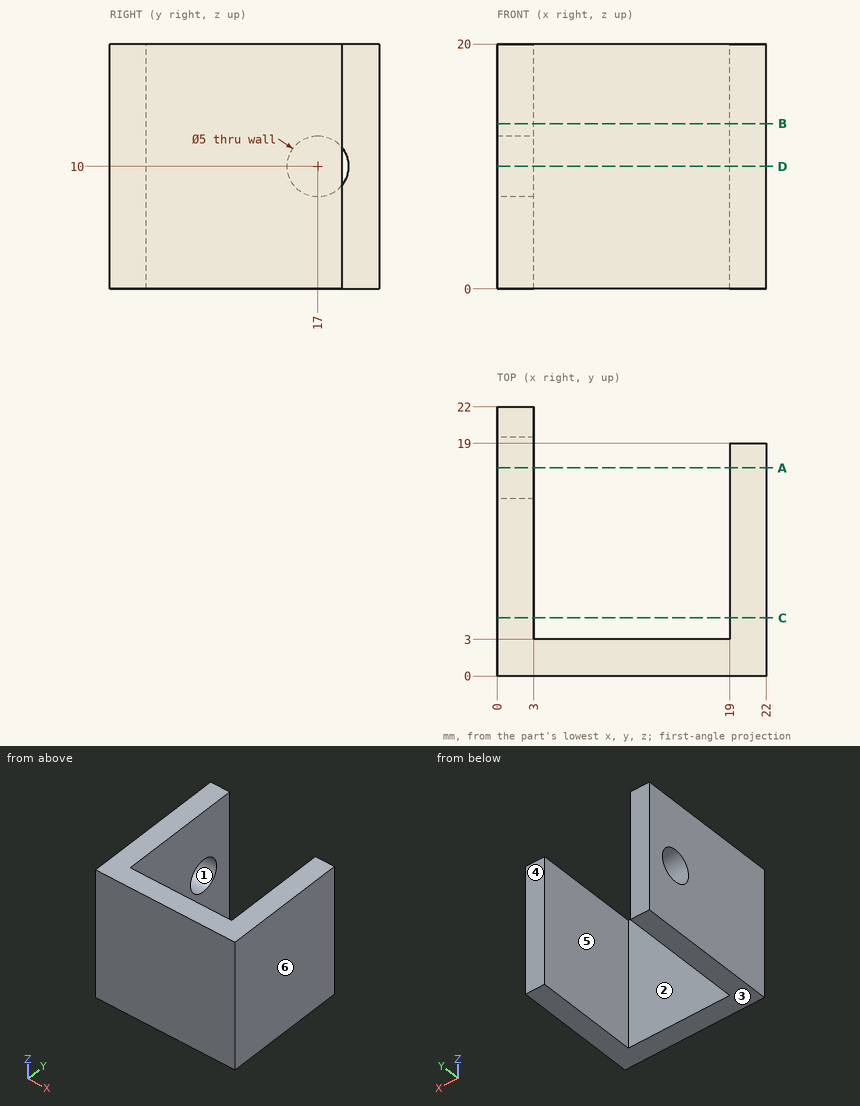
For this review, use the dimensioned drawing (mm, ordinates from the lowest corner) and the shaded views. A direction names the side the tool comes from. Round coordinates to 2 decimals unless told otherwise and drop trailing zeros. Write each loop counter-clockwise with the first axis right and the second up, starting at its lowest first coordinate (ties: lowest second). Pieces come first, ordered by that corner, then holes. Notation, with made-up numbers: M 35,-28.75 L 80,-28.75 A34 cw 80,2.25 Z; hole C 9,73.25 d3. An arc over 180 degrees is marked long. Answer as CSV lines item,"result". Start each with the question number.
Q1. Consider section B-B, the plane z = 13.5. Give the boundary of the cut face in (x, y).
Q2. Clearance check with flat-ended pins moving along their axes: P1, Ø5, axis at y = 13, z = 10.5, coming from the -X side; P2, Ø3.5, axis at x = 20, z = 12, coming from the +Y side; P3, Ø1.5, axis at x = 5, y = 10.5, coming from the +Z side; P4, Ø3, axis at x = 11, z = 15, coming from the +Y side. State where each tip first meets the part, or that it passes through.
Q3. Tool access review of the marked faces 1, 2 and 3: name each direction out of +Z, -Z, +X, -X, +Y, -Y from which nothing blocks a thin tool from reaching the whole face with its end or side.
Q4. The part is to be moulded in two halves that separate along X. For the marked faces 4, 5 and 6, say which applies: +X half, -X half, draft (parallel to the pull), parting line (faces both ways), or undercut.
Q5. Consider section A-A, the plane y = 17. Give the boundary of the cut face in (x, z), then the cut area to 3 significant figures.
Q6. Wall thickness on line 1 along Y through (x, z) = (1.75, 10); line 2 along X through (y, z) = (5.25, 1.5); line 3 along X through (y, z) = (19.5, 13): over which ranges is each line inside the solid? List them lowest first.
Q7. Consider section C-C, the plane y = 4.75. Give the boundary of the cut face in (x, z), then the cut area to 3 significant figures.
Q8. Consider section D-D, the plane z = 10. Give the boundary of the cut face in (x, y), then the cut area to 3 significant figures.
Result set:
1,outline,"M 0,0 L 22,0 L 22,19 L 19,19 L 19,3 L 3,3 L 3,22 L 0,22 Z"
2,P1,"stops at x = 0"
2,P2,"stops at y = 19"
2,P3,"passes through"
2,P4,"stops at y = 3"
3,face 1,"-X"
3,face 2,"+Z, -Z, +Y"
3,face 3,"-Z, +X, -X, +Y, -Y"
4,face 4,"draft"
4,face 5,"undercut"
4,face 6,"+X half"
5,outline,"M 0,0 L 3,0 L 3,7.5 L 0,7.5 Z; M 0,12.5 L 3,12.5 L 3,20 L 0,20 Z; M 19,0 L 22,0 L 22,20 L 19,20 Z"
5,area,"105 mm²"
6,line 1,"y = 0 to 14.5, 19.5 to 22"
6,line 2,"x = 0 to 3, 19 to 22"
6,line 3,"x = 0 to 3"
7,outline,"M 0,0 L 3,0 L 3,20 L 0,20 Z; M 19,0 L 22,0 L 22,20 L 19,20 Z"
7,area,"120 mm²"
8,outline,"M 0,0 L 22,0 L 22,19 L 19,19 L 19,3 L 3,3 L 3,14.5 L 0,14.5 Z; M 0,19.5 L 3,19.5 L 3,22 L 0,22 Z"
8,area,"156 mm²"
